CAD build for the part. Positions are in the model's coordinates, mm. Face numbers are marked on the shaded views. A direction names the side the tool comes from. Coordinates: 2 decimals unless noted, no trailing zeros. Order: outer loops, then holes, each group sorted by start corner. A loop starts at its lowest first (then second) coordinate and runs counter-clockwise, first axis right, second up. Notation, with made-up numbers: M -38.5,-19 L -3.5,-19 A30 cw -3.5,10 Z; hole C 73,-7.75 d1. An arc over 180 degrees is marked long. One line per item, written item: value.
from build123d import *

# Parameters (mm, degrees)
SKETCH1_W                      = 42
SKETCH1_H                      = 32
BOSS_EXTRUDE1_DEPTH            = 13
SKETCH2_W                      = 12
SKETCH2_H                      = 26
CUT_EXTRUDE1_DEPTH             = 33.929191193
SKETCH3_W                      = 12
SKETCH3_H                      = 26
CUT_EXTRUDE2_DEPTH             = 33.929191193
CUT_EXTRUDE3_DEPTH             = 33.929191193
SKETCH5_W                      = 4
SKETCH5_H                      = 13
F_6_5_6_5_DIAMETER_HOLE1_D     = 6.5
F_6_5_6_5_DIAMETER_HOLE1_DEPTH = 32
F_6_5_6_5_DIAMETER_HOLE2_D     = 6.5
FILLET1_R                      = 0.5


with BuildPart() as part:
    # Sketch1 → Boss-Extrude1 (new body)
    with BuildSketch(Plane(origin=(0, 0, 0), x_dir=(-1, 0, 0), z_dir=(0, 0, -1))):
        with Locations((0.285714286, -5.5)):
            Rectangle(SKETCH1_W, SKETCH1_H)
    extrude(amount=-BOSS_EXTRUDE1_DEPTH)

    # Sketch2 → Cut-Extrude1 (cut, through all)
    with BuildSketch(Plane.XY.offset(13)):
        with Locations((14.714285714, -2.5)):
            Rectangle(SKETCH2_W, SKETCH2_H)
    extrude(amount=-CUT_EXTRUDE1_DEPTH, mode=Mode.SUBTRACT)

    # Sketch3 → Cut-Extrude2 (cut, through all)
    with BuildSketch(Plane.XY.offset(13)):
        with Locations((-15.285714286, -2.5)):
            Rectangle(SKETCH3_W, SKETCH3_H)
    extrude(amount=-CUT_EXTRUDE2_DEPTH, mode=Mode.SUBTRACT)

    # Sketch4 → Cut-Extrude3 (cut, through all)
    with BuildSketch(Plane.XY.offset(13)):
        with BuildLine():
            Line((0.214285714, 10.5), (-0.785714286, 10.5))
            Line((-0.785714286, 10.5), (-0.785714286, 2.5))
            ThreePointArc((-0.785714286, 2.5), (-0.285714286, 2.531373033), (0.214285714, 2.5))
            Line((0.214285714, 2.5), (0.214285714, 10.5))
        make_face()
    extrude(amount=-CUT_EXTRUDE3_DEPTH, mode=Mode.SUBTRACT)

    # Sketch5 → Cut-Revolve1 (revolve, cut)
    with BuildSketch(Plane(origin=(0, -1.468626967, 0), x_dir=(1, 0, 0), z_dir=(0, 1, 0))):
        with Locations((1.714285714, -6.5)):
            Rectangle(SKETCH5_W, SKETCH5_H)
    revolve(axis=Axis((-0.285714286, -1.468626967, 0), (0, 0, 1)), mode=Mode.SUBTRACT)

    # Ø6.5 (6.5) Diameter Hole1
    with Locations(Plane(origin=(0, -21.5, 0), x_dir=(-1, 0, 0), z_dir=(0, -1, 0))):
        with Locations((-14.714285714, -6.749358536)):
            Hole(F_6_5_6_5_DIAMETER_HOLE1_D / 2, depth=F_6_5_6_5_DIAMETER_HOLE1_DEPTH)

    # Ø6.5 (6.5) Diameter Hole2 (through all)
    with Locations(Plane(origin=(0, -15.5, 0), x_dir=(1, 0, 0), z_dir=(0, 1, 0))):
        with Locations((-15.285714286, -6.749358536)):
            Hole(F_6_5_6_5_DIAMETER_HOLE2_D / 2)

    # Fillet1
    fillet1_edges = [part.edges().sort_by_distance(p)[0] for p in [
        (8.714285714, -15.5, 6.5),
        (-9.285714286, -15.5, 6.5),
    ]]
    fillet(fillet1_edges, radius=FILLET1_R)


solid = part.part
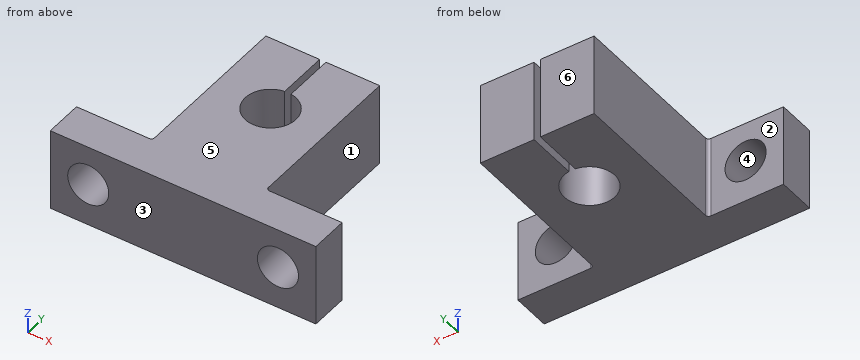
Q1. Slice it at D-D (y = -18). List the corners of the cut face in (x, z).
Recorded:
outline: M -21.29,0 L 20.71,0 L 20.71,13 L -21.29,13 Z; hole C -15.29,6.75 d6.5; hole C 14.71,6.75 d6.5
Q2. Slice it at B-B (z = 10.5). List the corners of the cut face in (x, y), plus the area to 3 significant figures.
Recorded:
outline: M -21.29,-21.5 L 20.71,-21.5 L 20.71,-15.5 L 9.21,-15.5 A0.5 cw 8.71,-15 L 8.71,10.5 L 0.21,10.5 L 0.21,2.5 A4 cw long -0.79,2.5 L -0.79,10.5 L -9.29,10.5 L -9.29,-15 A0.5 cw -9.79,-15.5 L -21.29,-15.5 Z
area: 662 mm^2
Q3. Pin check, flat tips, straight feed: pin 1 Ø1.5 at (y, z) = (-13.5, 2) entering from -X; pin 2 Ø3.5 at (x, z) = (-15.5, 8) entering from +Y; pin 3 Ø6.5 at (y, z) = (5.5, 8.5) entering from +X; pin 4 Ø3.5 at (x, z) = (16, 4) entering from +Y. Stop position of each tip, or through.
Recorded:
pin 1: stops at x = -9.29
pin 2: passes through
pin 3: stops at x = 8.71
pin 4: stops at y = -15.5
Q4. Mould opens along Z. For the marked faces 4, 5 and 6 say: released by +Z, released by -Z, zero draft, split by the parting line, or undercut.
Recorded:
face 4: undercut
face 5: released by +Z
face 6: zero draft
Q5. Slice it at A-A (y = 3). List the corners of the cut face in (x, z), plus the area to 3 significant figures.
Recorded:
outline: M -9.29,0 L -0.79,0 L -0.79,13 L -9.29,13 Z; M 0.21,0 L 8.71,0 L 8.71,13 L 0.21,13 Z
area: 221 mm^2
Q6. Which spindle directions (+Z, -Z, +X, -X, +Y, -Y) get a long thin tool onto all of the face, cutting with end or side? Do the marked faces 1, 2 and 3. Say none if no direction does.
Recorded:
face 1: +Z, -Z, +X, +Y
face 2: +Z, -Z, -X, +Y
face 3: +Z, -Z, +X, -X, -Y
Q7. Slice it at C-C (x = -2.5). List the corners of the cut face in (y, z), plus the area to 3 significant figures.
Recorded:
outline: M -21.5,0 L -4.8,0 L -4.8,13 L -21.5,13 Z; M 1.86,0 L 10.5,0 L 10.5,13 L 1.86,13 Z
area: 329 mm^2
Q8. Drill centre lines: line 1 along X through (y, z) = (5.5, 2.25); line 2 along X through (y, z) = (-20, 8.5); line 3 along Y through (x, z) = (2, 2). Where is each one in solid material? Low to high.
Recorded:
line 1: x = -9.29 to -0.79, 0.21 to 8.71
line 2: x = -21.29 to -18.02, -12.55 to 11.98, 17.45 to 20.71
line 3: y = -21.5 to -4.75, 1.81 to 10.5
